Work out the finished part from the listing and answer in its coordinate system (mm). Round coordinates to 2 decimals unless told otherwise and drop trailing zeros. Write each loop counter-clockwise with the first axis right and the second up, starting at its lowest first coordinate (ties: lowest second). Pieces come first, ordered by that corner, then holes. Notation, with made-up numbers: (31, 68.5) -> (69, 68.5) arc R7 ccw to (69, 75.5) -> close; hole circle Ø10 at (29.25, 19.25). An arc over 180 degrees is marked (long way). Answer as a JSON object with one key per item and string values. Group by question number.
from build123d import *

# Parameters (mm, degrees)
SKETCH1_R             = 5
BOSS_EXTRUDE1_DEPTH   = 25
SKETCH2_W             = 5
SKETCH2_H             = 15
BOSS_EXTRUDE2_DEPTH   = 5
SKETCH3_W             = 5
SKETCH3_H             = 15
BOSS_EXTRUDE3_DEPTH   = 2.5
SKETCH5_W             = 5
SKETCH5_H             = 15
BOSS_EXTRUDE5_DEPTH   = 2.5
BOSS_EXTRUDE6_START   = 25
SKETCH6_R             = 5
BOSS_EXTRUDE6_DEPTH   = 25
SKETCH7_W             = 5
SKETCH7_H             = 15
BOSS_EXTRUDE7_DEPTH   = 5
F_5_0MM_DOWEL_HOLE1_D = 5
BOSS_EXTRUDE8_START   = 20
SKETCH14_R            = 5
BOSS_EXTRUDE8_DEPTH   = 20
SKETCH15_R            = 5
BOSS_EXTRUDE9_DEPTH   = 20


with BuildPart() as part:
    # Sketch1 → Boss-Extrude1 (new body)
    with BuildSketch(Plane.XY):
        with Locations(Location((0, 0, 0), (0, 0, 180))):
            Circle(SKETCH1_R)
    extrude(amount=BOSS_EXTRUDE1_DEPTH)

    # Sketch2 → Boss-Extrude2 (add)
    with BuildSketch(Plane.XY.offset(25)):
        Rectangle(SKETCH2_W, SKETCH2_H)
    extrude(amount=-BOSS_EXTRUDE2_DEPTH)

    # Sketch3 → Boss-Extrude3 (add)
    with BuildSketch(Plane(origin=(0, 0, 0), x_dir=(-1, 0, 0), z_dir=(0, 0, -1))):
        Rectangle(SKETCH3_W, SKETCH3_H)
    extrude(amount=-BOSS_EXTRUDE3_DEPTH)

    # Sketch5 → Boss-Extrude5 (add)
    with BuildSketch(Plane(origin=(0, 0, 0), x_dir=(-1, 0, 0), z_dir=(0, 0, -1))):
        Rectangle(SKETCH5_W, SKETCH5_H)
    extrude(amount=BOSS_EXTRUDE5_DEPTH)

    # Sketch6 → Boss-Extrude6 (add)
    with BuildSketch(Plane(origin=(0, 0, 0), x_dir=(-1, 0, 0), z_dir=(0, 0, -1)).offset(BOSS_EXTRUDE6_START)):
        Circle(SKETCH6_R)
    extrude(amount=-BOSS_EXTRUDE6_DEPTH)

    # Sketch7 → Boss-Extrude7 (add)
    with BuildSketch(Plane(origin=(0, 0, -25), x_dir=(-1, 0, 0), z_dir=(0, 0, -1))):
        Rectangle(SKETCH7_W, SKETCH7_H)
    extrude(amount=-BOSS_EXTRUDE7_DEPTH)

    # Ø5.0mm Dowel Hole1 (through all)
    with Locations(Plane.XY.offset(25)):
        with Locations((0, 0)):
            Hole(F_5_0MM_DOWEL_HOLE1_D / 2)

    # Sketch14 → Boss-Extrude8 (add)
    with BuildSketch(Plane(origin=(0, 0, -25), x_dir=(-1, 0, 0), z_dir=(0, 0, -1)).offset(BOSS_EXTRUDE8_START)):
        Circle(SKETCH14_R)
    extrude(amount=-BOSS_EXTRUDE8_DEPTH)

    # Sketch15 → Boss-Extrude9 (add)
    with BuildSketch(Plane.XY.offset(25)):
        with Locations(Location((0, 0, 0), (0, 0, 180))):
            Circle(SKETCH15_R)
    extrude(amount=BOSS_EXTRUDE9_DEPTH)


solid = part.part
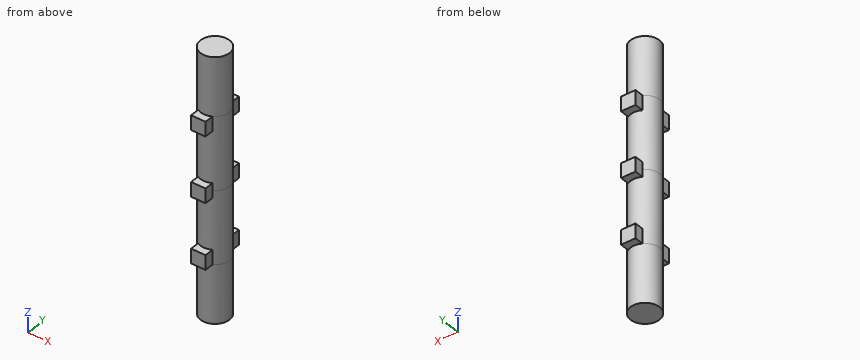
1) A cutting plane is placed at C-C on z = 1. Determine the outline of the cut face in (x, y).
2) A cutting plane is placed at A-A on y = 6.5. Determine the outline of the cut face in (x, z).
3) A cutting plane is placed at B-B on y = 0. Determine the outline of the cut face in (x, z).
4) Each of these flat-tipped pins is pushed along its axis until it touches: P1, Ø3.5, axis at y = 6, z = -23, coming from the -X side; P2, Ø1.6, axis at y = -5, z = -23.5, coming from the +X side; P3, Ø1.6, axis at y = -5.5, z = 0, coming from the +X side; P4, Ø3.5, axis at x = -1, y = 6, coming from the -Z side. Where does it stop, or does it pass through?
5) Straight lines are drawn through the part: L1, parallel to Z at x = 0, y = 6.5; L2, parallel to Y at x = 0, z = 11.5; L3, parallel to Z at x = 0.25, y = 1. For each, find the intervals that lie inside material, in ascending order.
Established:
{
 "1": {"outline": "(-2.5, -7.5) -> (2.5, -7.5) -> (2.5, -4.33) arc R5 ccw to (2.5, 4.33) -> (2.5, 7.5) -> (-2.5, 7.5) -> (-2.5, 4.33) arc R5 ccw to (-2.5, -4.33) -> close; hole circle Ø5 at (0, 0)"},
 "2": {"outline": "(-2.5, -25) -> (2.5, -25) -> (2.5, -20) -> (-2.5, -20) -> close; (-2.5, -2.5) -> (2.5, -2.5) -> (2.5, 2.5) -> (-2.5, 2.5) -> close; (-2.5, 20) -> (2.5, 20) -> (2.5, 25) -> (-2.5, 25) -> close"},
 "3": {"outline": "(-5, -45) -> (5, -45) -> (5, 45) -> (-5, 45) -> close; hole (-2.5, -25) -> (2.5, -25) -> (2.5, 25) -> (-2.5, 25) -> close"},
 "4": {"P1": "stops at x = -2.63", "P2": "stops at x = 2.71", "P3": "stops at x = 2.5", "P4": "stops at z = -45"},
 "5": {"L1": "z = -25 to -20, -2.5 to 2.5, 20 to 25", "L2": "y = -5 to -2.5, 2.5 to 5", "L3": "z = -45 to -25, 25 to 45"}
}
